Part print with two shaded views. Sizes in mm from the minimum x, y, z corner. Give positions to 0.01 mm unless a question says otherwise; leave off trailing zeros. Order: outer loops, then holes, each group sorted by start corner. A loop starts at its lowest first (then second) coordinate and runs counter-clockwise, first axis right, second up. Notation, with made-up numbers: M 65,33.25 L 114,33.25 A19 cw 114,65.25 Z; hole C 35.25,64 d7. An arc over 180 degrees is marked long. Return JSON: item names as keys, results as strings.
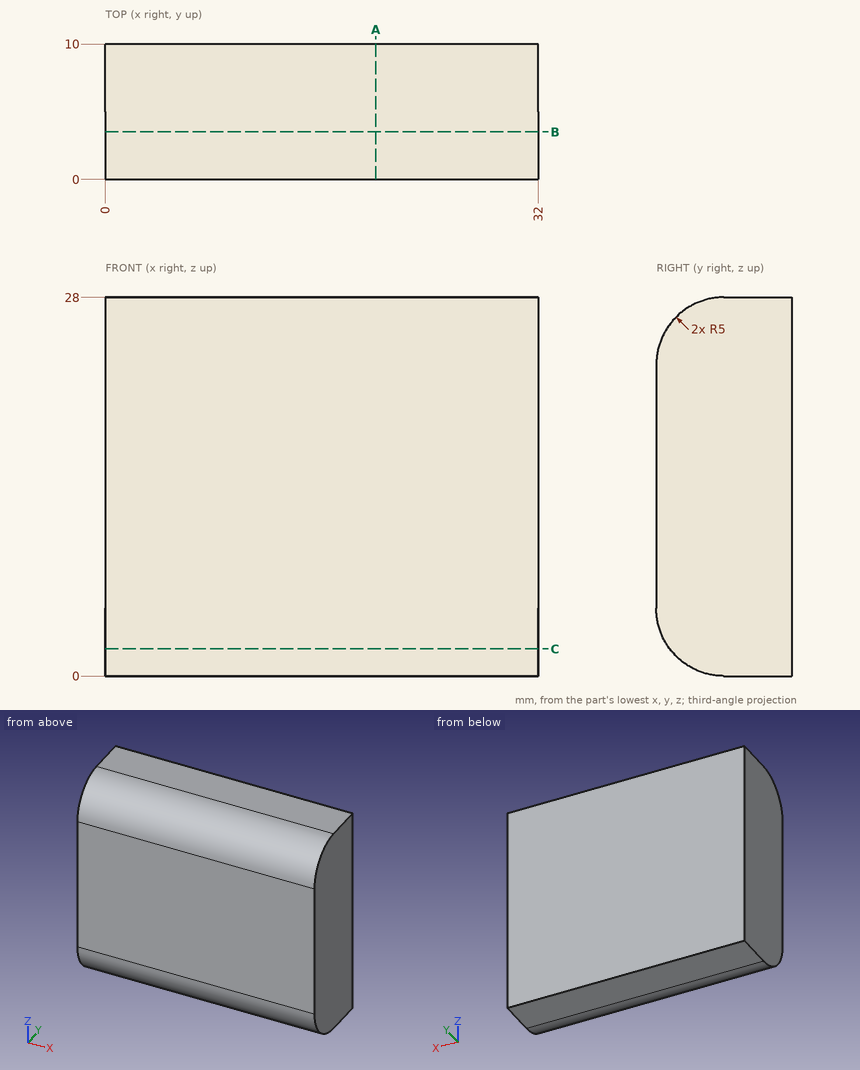
Q1. Band-saw the part on C-C (z = 2). Give the cut face in (x, y), then the cut area to 3 significant figures.
Established:
{"outline": "M 0,1 L 32,1 L 32,10 L 0,10 Z", "area": "288 mm²"}
Q2. Band-saw the part on A-A (x = 20). Give the cut face in (y, z), then the cut area to 3 significant figures.
Established:
{"outline": "M 0,5 A5 ccw 5,0 L 10,0 L 10,28 L 5,28 A5 ccw 0,23 Z", "area": "269 mm²"}
Q3. Band-saw the part on B-B (y = 3.5). Give the cut face in (x, z).
Established:
{"outline": "M 0,0.23 L 32,0.23 L 32,27.77 L 0,27.77 Z"}
Q4. Pin check, flat tip, straight feed: pin 1 (6 mm diameter, centred on x = 25.5, z = 5.5, fed in from -Y). Stop position of the tip, or through.
Established:
{"pin 1": "stops at y = 0"}
Q5. Probe line 1 along Z through (x, y) = (31.5, 3); line 2 along Y through (x, z) = (14, 24); line 3 along Z through (x, y) = (7.5, 2.75). List the from-to ranges inside material, lowest first.
Established:
{"line 1": "z = 0.42 to 27.58", "line 2": "y = 0.1 to 10", "line 3": "z = 0.53 to 27.47"}
